```python
from build123d import *

# Parameters (mm, degrees)
F1_DEPTH = 12.7


with BuildPart() as f1:
    # F0 (on Top) → F1 (new body)
    with BuildSketch(Plane.XY):
        with BuildLine():
            ThreePointArc((7.045173, -2.57207), (7.385418, -1.305987), (7.5, 0))
            ThreePointArc((7.5, 0), (5.123577, 5.47713), (-0.499722, 7.483333))
            ThreePointArc((-0.499722, 7.483333), (-0.99833, 7.433259), (-1.492481, 7.35))
            ThreePointArc((-1.492481, 7.35), (-6.992258, 2.712624), (-6.058809, -4.420501))
            ThreePointArc((-6.058809, -4.420501), (-5.938513, -4.580836), (-5.813975, -4.7379))
            ThreePointArc((-5.813975, -4.7379), (0.948225, -7.439817), (6.816519, -3.128109))
            ThreePointArc((6.816519, -3.128109), (6.93642, -2.852382), (7.045173, -2.57207))
        make_face()
        with BuildLine():
            ThreePointArc((-1.492481, 7.35), (-0.99833, 7.433259), (-0.499722, 7.483333))
            ThreePointArc((-0.499722, 7.483333), (-0.359398, 7.847611), (0, 8))
            ThreePointArc((0, 8), (1.5, 9.5), (0, 11))
            ThreePointArc((0, 11), (-0.5, 11.5), (0, 12))
            ThreePointArc((0, 12), (1.5, 13.5), (0, 15))
            ThreePointArc((0, 15), (-0.5, 15.5), (0, 16))
            ThreePointArc((0, 16), (1.5, 17.5), (0, 19))
            ThreePointArc((0, 19), (-0.5, 19.5), (0, 20))
            ThreePointArc((0, 20), (1.5, 21.5), (0, 23))
            ThreePointArc((0, 23), (-0.5, 23.5), (0, 24))
            ThreePointArc((0, 24), (1.5, 25.5), (0, 27))
            Line((0, 27), (0, 26))
            ThreePointArc((0, 26), (0.5, 25.5), (0, 25))
            ThreePointArc((0, 25), (-1.5, 23.5), (0, 22))
            ThreePointArc((0, 22), (0.5, 21.5), (0, 21))
            ThreePointArc((0, 21), (-1.5, 19.5), (0, 18))
            ThreePointArc((0, 18), (0.5, 17.5), (0, 17))
            ThreePointArc((0, 17), (-1.5, 15.5), (0, 14))
            ThreePointArc((0, 14), (0.5, 13.5), (0, 13))
            ThreePointArc((0, 13), (-1.5, 11.5), (0, 10))
            ThreePointArc((0, 10), (0.5, 9.5), (0, 9))
            ThreePointArc((0, 9), (-1.11243, 8.506231), (-1.492481, 7.35))
        make_face()
        with BuildLine():
            ThreePointArc((7.621024, -4.4), (7.735118, -3.359387), (7.045173, -2.57207))
            ThreePointArc((7.045173, -2.57207), (6.93642, -2.852382), (6.816519, -3.128109))
            ThreePointArc((6.816519, -3.128109), (7.166926, -3.553095), (7.101408, -4.1))
            ThreePointArc((7.101408, -4.1), (7.577241, -5.875833), (9.353074, -5.4))
            ThreePointArc((9.353074, -5.4), (10.309292, -5.143782), (10.56551, -6.1))
            ThreePointArc((10.56551, -6.1), (11.041343, -7.875833), (12.817176, -7.4))
            ThreePointArc((12.817176, -7.4), (13.773394, -7.143782), (14.029612, -8.1))
            ThreePointArc((14.029612, -8.1), (14.505445, -9.875833), (16.281278, -9.4))
            ThreePointArc((16.281278, -9.4), (17.237495, -9.143782), (17.493713, -10.1))
            ThreePointArc((17.493713, -10.1), (17.969546, -11.875833), (19.745379, -11.4))
            ThreePointArc((19.745379, -11.4), (20.701597, -11.143782), (20.957815, -12.1))
            ThreePointArc((20.957815, -12.1), (21.433648, -13.875833), (23.209481, -13.4))
            Line((23.209481, -13.4), (22.689866, -13.1))
            ThreePointArc((22.689866, -13.1), (21.733648, -13.356218), (21.47743, -12.4))
            ThreePointArc((21.47743, -12.4), (21.001597, -10.624167), (19.225764, -11.1))
            ThreePointArc((19.225764, -11.1), (18.269546, -11.356218), (18.013328, -10.4))
            ThreePointArc((18.013328, -10.4), (17.537495, -8.624167), (15.761662, -9.1))
            ThreePointArc((15.761662, -9.1), (14.805445, -9.356218), (14.549227, -8.4))
            ThreePointArc((14.549227, -8.4), (14.073394, -6.624167), (12.297561, -7.1))
            ThreePointArc((12.297561, -7.1), (11.341343, -7.356218), (11.085125, -6.4))
            ThreePointArc((11.085125, -6.4), (10.609292, -4.624167), (8.833459, -5.1))
            ThreePointArc((8.833459, -5.1), (7.877241, -5.356218), (7.621024, -4.4))
        make_face()
        with BuildLine():
            ThreePointArc((-5.813975, -4.7379), (-5.938513, -4.580836), (-6.058809, -4.420501))
            ThreePointArc((-6.058809, -4.420501), (-6.681558, -4.527989), (-7.188011, -4.15))
            ThreePointArc((-7.188011, -4.15), (-8.827241, -3.71077), (-9.266472, -5.35))
            ThreePointArc((-9.266472, -5.35), (-9.559292, -6.44282), (-10.652112, -6.15))
            ThreePointArc((-10.652112, -6.15), (-12.291343, -5.71077), (-12.730573, -7.35))
            ThreePointArc((-12.730573, -7.35), (-13.023394, -8.44282), (-14.116214, -8.15))
            ThreePointArc((-14.116214, -8.15), (-15.755445, -7.71077), (-16.194675, -9.35))
            ThreePointArc((-16.194675, -9.35), (-16.487495, -10.44282), (-17.580316, -10.15))
            ThreePointArc((-17.580316, -10.15), (-19.219546, -9.71077), (-19.658777, -11.35))
            ThreePointArc((-19.658777, -11.35), (-19.951597, -12.44282), (-21.044417, -12.15))
            ThreePointArc((-21.044417, -12.15), (-22.683648, -11.71077), (-23.122878, -13.35))
            Line((-23.122878, -13.35), (-22.776468, -13.15))
            ThreePointArc((-22.776468, -13.15), (-22.483648, -12.05718), (-21.390827, -12.35))
            ThreePointArc((-21.390827, -12.35), (-19.751597, -12.78923), (-19.312367, -11.15))
            ThreePointArc((-19.312367, -11.15), (-19.019546, -10.05718), (-17.926726, -10.35))
            ThreePointArc((-17.926726, -10.35), (-16.287495, -10.78923), (-15.848265, -9.15))
            ThreePointArc((-15.848265, -9.15), (-15.555445, -8.05718), (-14.462624, -8.35))
            ThreePointArc((-14.462624, -8.35), (-12.823394, -8.78923), (-12.384163, -7.15))
            ThreePointArc((-12.384163, -7.15), (-12.091343, -6.05718), (-10.998523, -6.35))
            ThreePointArc((-10.998523, -6.35), (-9.359292, -6.78923), (-8.920062, -5.15))
            ThreePointArc((-8.920062, -5.15), (-8.627241, -4.05718), (-7.534421, -4.35))
            ThreePointArc((-7.534421, -4.35), (-6.759123, -4.920615), (-5.813975, -4.7379))
        make_face()
    extrude(amount=F1_DEPTH)


solid = f1.part
```
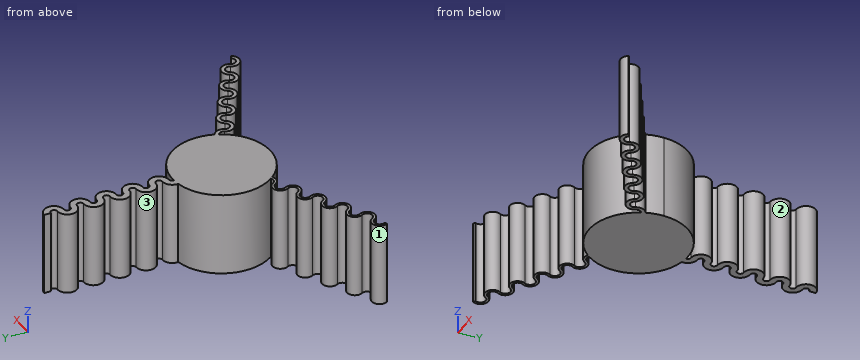
The model under review builds one solid part; all positions refer to its coordinate system, in mm. Face numbers are marked on the shaded views. Give positions to 0.01 mm unless a question says otherwise; leave off trailing zeros. Order: outer loops, then holes, each group sorted by start corner. A loop starts at its lowest first (then second) coordinate and runs counter-clockwise, first axis right, second up. Notation, with made-up numbers: (-27, 58) - (1, 58) arc R17 ccw to (1, 76) - close; hole circle Ø7 at (87.25, 33). An arc over 180 degrees is marked (long way). Use CSV: the item, a comma, the result in double quotes. Start each with the question number.
Q1. To check wall thickness, follow line 1 along X through (y, z) = (-11, 10); line 2 along Y through (x, z) = (-10, 3.25); line 3 along X through (y, z) = (-3.5, 4.75). State the ranges of each line that lie inside material, in increasing order. Write a range as [from, to].
Q2. Clearance check with flat-ended pins moving along their axes: pin 1 Ø5 at (x, z) = (18.5, 5) entering from -Y; pin 2 Ø5 at (x, z) = (-9.5, 4) entering from -Y; pin 3 Ø3 at (y, z) = (14, 6) entering from -X. State where each tip first meets the part, or that it passes through.
Q3. The part is to be moulded in two halves that separate along X. For the marked faces 1, 2 and 3, say which applies: +X half, -X half, draft (parallel to the pull), parting line (faces both ways), or undercut.
Q4. We need section A-A, the plane y = -1. Write out the cut boundary in (x, z).
Outcome:
1,line 1,"x = [-19.79, -19.38], [17.34, 17.97], [19.29, 21.41]"
1,line 2,"y = [-6.95, -6.55]"
1,line 3,"x = [-6.63, 6.63], [7.15, 7.77]"
2,pin 1,"stops at y = -13.47"
2,pin 2,"stops at y = -6.95"
2,pin 3,"stops at x = -1.5"
3,face 1,"undercut"
3,face 2,"+X half"
3,face 3,"-X half"
4,outline,"(-7.43, 0) - (7.43, 0) - (7.43, 12.7) - (-7.43, 12.7) - close"
